Answer from the drawing. Dimensions are ordinates in mm from the lowest x, y and z of the part. Coordinates: 2 decimals unless noted, no trailing zeros. Order: outer loops, then holes, each group sorted by start corner. A loop starts at its lowest first (then second) coordinate and runs counter-clockwise, first axis right, second up. Notation, with made-up numbers: (19.5, 2) -> (50.5, 2) arc R9 ccw to (50.5, 7) -> close; hole circle Ø10 at (60.5, -14.5). An arc over 180 degrees is marked (long way). Answer in a Markdown table with one row per item.
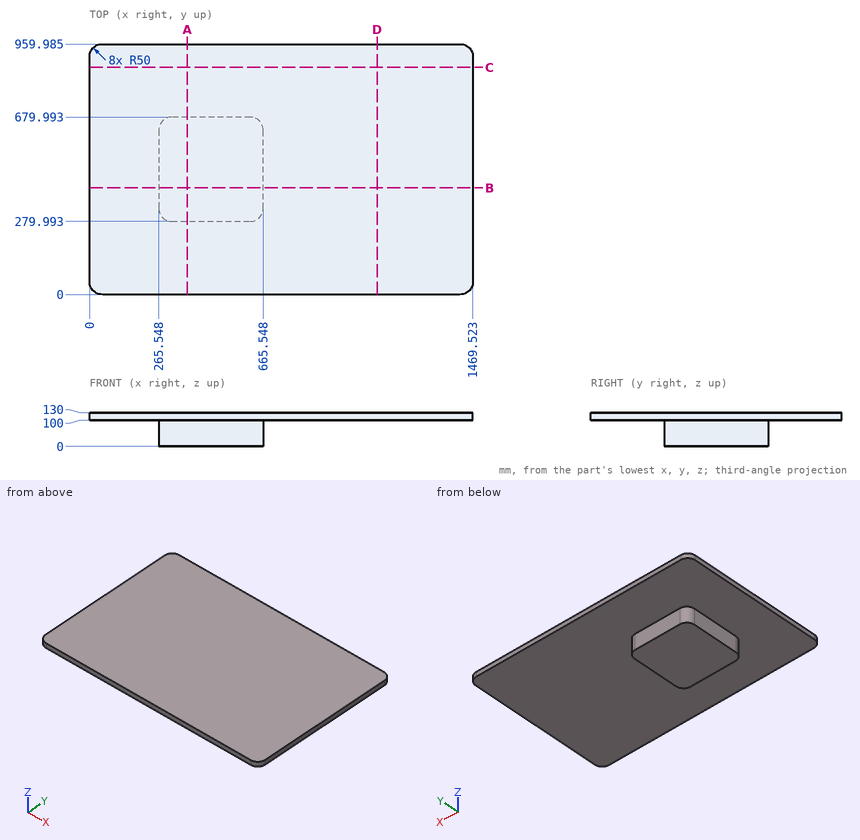
Q1. The part is cut by section C-C (y = 870.5). Write down the section's boundary in (x, z), then the cut area to 3 significant figures.
Outcome:
| item | result |
|---|---|
| outline | (0, 100) -> (1469.52, 100) -> (1469.52, 130) -> (0, 130) -> close |
| area | 44,100 mm² |
Q2. The part is cut by section A-A (x = 375). Write down the section's boundary in (y, z) (1 decimal).
Outcome:
| item | result |
|---|---|
| outline | (0, 100) -> (280, 100) -> (280, 0) -> (680, 0) -> (680, 100) -> (960, 100) -> (960, 130) -> (0, 130) -> close |
Q3. The part is cut by section D-D (x = 1102.5). Write down the section's boundary in (y, z) (1 decimal).
Outcome:
| item | result |
|---|---|
| outline | (0, 100) -> (960, 100) -> (960, 130) -> (0, 130) -> close |
Q4. Consider line 1 (X direction, y = 338, z = 14.5); line 2 (Y direction, x = 381, z = 82); line 3 (X direction, y = 633.5, z = 15.5) (1 decimal). Determine where each line is inside the solid, lowest interval first.
Outcome:
| item | result |
|---|---|
| line 1 | 265.55 to 665.55 |
| line 2 | 279.99 to 679.99 |
| line 3 | 265.7 to 665.4 |
Q5. Given pin 1 (8 mm diameter, centred on y = 275.5, z = 64, fed in from +X); pin 2 (12 mm diameter, centred on x = 286.5, z = 23.5, fed in from +Y), each flat-ended and moving along its own axis, determine where each tip first touches the part or whether it passes through.
Outcome:
| item | result |
|---|---|
| pin 1 | through |
| pin 2 | y = 674.36 |
Q6. The part is cut by section B-B (y = 408.5). Write down the section's boundary in (x, z).
Outcome:
| item | result |
|---|---|
| outline | (0, 100) -> (265.55, 100) -> (265.55, 0) -> (665.55, 0) -> (665.55, 100) -> (1469.52, 100) -> (1469.52, 130) -> (0, 130) -> close |
